```python
from build123d import *

# Parameters (mm, degrees)
SKETCH1_W           = 25
SKETCH1_H           = 25
BOSS_EXTRUDE1_DEPTH = 10
BOSS_EXTRUDE1_DRAFT = -11
CAVITY1_OUTLINE_W   = 18.62330315
CAVITY1_OUTLINE_H   = 18.62330315
CAVITY1_OUTLINE_W_2 = 14.62330315
CAVITY1_OUTLINE_H_2 = 14.62330315
CAVITY1_DEPTH       = 5.060188455
CAVITY1_DRAFT       = 12


# Read off the part's stored shape, not the designer's step: Cavity1
with BuildPart() as part:
    # Sketch1 → Boss-Extrude1 (with draft: the straight prism first)
    with BuildSketch(Plane(origin=(0, 0, 0), x_dir=(1, 0, 0), z_dir=(0, 1, 0))):
        with Locations((-4.792449363, -1.137627393)):
            Rectangle(SKETCH1_W, SKETCH1_H)
    extrude(amount=BOSS_EXTRUDE1_DEPTH)
    # Boss-Extrude1: the draft: its side faces are tilted about the plane it starts from
    boss_extrude1_sides = [part.faces().sort_by_distance(p)[0] for p in [
        (-17.292449363, 5, 1.137627393),
        (-4.792449363, 5, 13.637627393),
        (7.707550637, 5, 1.137627393),
        (-4.792449363, 5, -11.362372607),
    ]]
    draft(boss_extrude1_sides, Plane(origin=(0, 0, 0), x_dir=(1, 0, 0), z_dir=(0, 1, 0)), BOSS_EXTRUDE1_DRAFT)


with BuildPart() as cavity1_tool:
    # Cavity1 outline → Cavity1 (with draft: the straight prism first)
    with BuildSketch(Plane(origin=(0, 5.060188455, 0), x_dir=(1, 0, 0), z_dir=(0, 1, 0))):
        with Locations((-4.792449363, -1.137627393)):
            Rectangle(CAVITY1_OUTLINE_W, CAVITY1_OUTLINE_H)
        with Locations((-4.792449363, -1.137627393)):
            Rectangle(CAVITY1_OUTLINE_W_2, CAVITY1_OUTLINE_H_2, mode=Mode.SUBTRACT)
    extrude(amount=-CAVITY1_DEPTH)
    # Cavity1: the draft: its side faces are tilted about the plane it starts from
    cavity1_sides = [cavity1_tool.faces().sort_by_distance(p)[0] for p in [
        (-14.104100938, 2.530094227, 1.137627393),
        (-4.792449363, 2.530094227, 10.449278968),
        (4.519202212, 2.530094227, 1.137627393),
        (-4.792449363, 2.530094227, -8.174024182),
        (2.519202212, 2.530094227, 1.137627393),
        (-4.792449363, 2.530094227, 8.449278968),
        (-12.104100938, 2.530094227, 1.137627393),
        (-4.792449363, 2.530094227, -6.174024182),
    ]]
    draft(cavity1_sides, Plane(origin=(0, 5.060188455, 0), x_dir=(1, 0, 0), z_dir=(0, 1, 0)), CAVITY1_DRAFT)


with BuildPart() as part_1:
    add(part.part)

    # Cavity1: cut by cavity1_tool
    add(cavity1_tool.part, mode=Mode.SUBTRACT)


solid = part_1.part
```
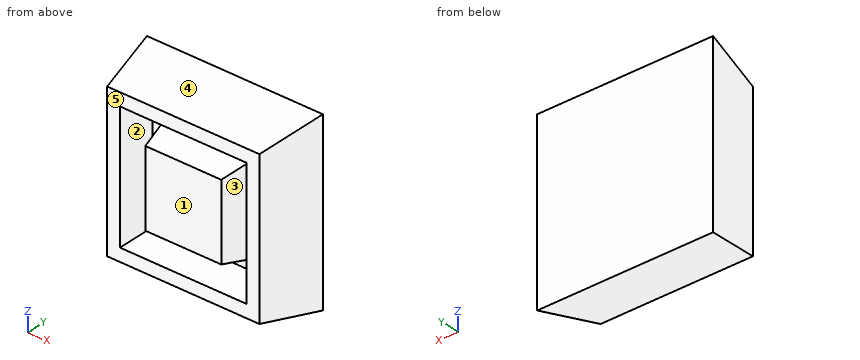
The model under review builds one solid part; all positions refer to its coordinate system, in mm. Face numbers are marked on the shaded views. A direction names the side the tool comes from. Round coordinates to 2 decimals unless told otherwise and drop trailing zeros. Loops run counter-clockwise (first coordinate to the right, second up) from the corner with the lowest first, then second, coordinate; pieces in that order, holes last. Notation, with made-up numbers: M 48.5,-3.5 L 68.5,-3.5 A27 ccw 68.5,14.5 Z; hole C -27.75,58 d11. An arc over 180 degrees is marked long. Put each result on its own line as item: value.
Q1. For pin 1 (1.5 mm diameter, centred on y = 4, z = 11.5, fed in from +X); pin 2 (3 mm diameter, centred on y = 1.5, z = 5, fed in from +X); pin 3 (1.5 mm diameter, centred on x = 6, y = 4, fed in from +Z), all flat-tipped, find the tip position at first contact; note any pin that passes through.
Result set:
pin 1: stops at x = 8.63
pin 2: stops at x = 8.29
pin 3: stops at z = 14.56
Q2. Machinability: for the marked faces 1 and 2, which of the approach directions +Z, -Z, +X, -X, +Y, -Y give a long, thin tool a straight path to every point of the face, cutting with its end or side? Answer none if there is none.
Result set:
face 1: +Z, -Z, +X, -X, -Y
face 2: -Y
Q3. To check wall thickness, follow L1, parallel to X at y = 5, z = 1; L2, parallel to Z at x = 0.75, y = 1.5; L3, parallel to Y at x = -1.25, z = -7.5. State the ranges of each line that lie inside material, in increasing order.
Result set:
L1: x = -18.26 to -14.12, -12.09 to 2.51, 4.53 to 8.68
L2: z = -11.65 to -8.93, -5.42 to 7.69, 11.21 to 13.93
L3: y = 5.06 to 10
Q4. Consider section A-A, the plane y = 4. Give the boundary of the cut face in (x, z).
Result set:
outline: M -18.07,-12.14 L 8.49,-12.14 L 8.49,14.42 L -18.07,14.42 Z; M -11.88,-5.95 L 2.29,-5.95 L 2.29,8.22 L -11.88,8.22 Z; hole M -14.33,-8.4 L 4.74,-8.4 L 4.74,10.67 L -14.33,10.67 Z
Q5. Consider section D-D, the plane z = -7. Give the boundary of the cut face in (x, y).
Result set:
outline: M -19.24,10 L -17.29,0 L -15.18,0 L -14.1,5.06 L 4.52,5.06 L 5.59,0 L 7.71,0 L 9.65,10 Z
Q6. Consider section C-C, the plane x = -5. Give the boundary of the cut face in (y, z), then the cut area to 3 significant figures.
Result set:
outline: M 0,-11.36 L 10,-13.31 L 10,15.58 L 0,13.64 L 0,11.52 L 5.06,10.45 L 5.06,8.45 L 0,7.37 L 0,-5.1 L 5.06,-6.17 L 5.06,-8.17 L 0,-9.25 Z
area: 238 mm²
Q7. Mouldability with a two-part tool opening along Z and no side actions: class the marked faces 3, 4 and 5 as released by +Z, released by -Z, zero draft, split by the parting line, or undercut.
Result set:
face 3: undercut
face 4: released by +Z
face 5: zero draft
Q8. Consider section B-B, the plane z = -1. Give the boundary of the cut face in (x, y).
Result set:
outline: M -19.24,10 L -17.29,0 L -15.18,0 L -14.1,5.06 L -12.1,5.06 L -11.03,0 L 1.44,0 L 2.52,5.06 L 4.52,5.06 L 5.59,0 L 7.71,0 L 9.65,10 Z
